```python
from build123d import *

# Parameters (mm, degrees)
EXTRUDE_1_DEPTH     = 100
CUT_EXTRUDE_1_DEPTH = 100


with BuildPart() as part:
    # Model → Бобышка-Вытянуть1 (new body)
    with BuildSketch(Plane.XY):
        with BuildLine():
            Line((-12.5, 11.1), (-12, 11.1))
            Line((-12, 11.1), (-12, 10.6))
            Line((-12, 10.6), (-11.1, 10.6))
            Line((-11.1, 10.6), (-11.1, 13.5))
            Line((-11.1, 13.5), (-9.3, 13.5))
            Line((-9.3, 13.5), (-6.8, 11))
            Line((-6.8, 11), (-6.8, 4))
            Line((-6.8, 4), (-9.3, 1.5))
            Line((-9.3, 1.5), (-11.1, 1.5))
            Line((-11.1, 1.5), (-11.1, 4.4))
            Line((-11.1, 4.4), (-12, 4.4))
            Line((-12, 4.4), (-12, 3.9))
            Line((-12, 3.9), (-12.5, 3.9))
            Line((-12.5, 3.9), (-12.5, 1.5))
            ThreePointArc((-12.5, 1.5), (-12.060660172, 0.439339828), (-11, 0))
            Line((-11, 0), (26.7, 0))
            Line((26.7, 0), (26.7, 1.3))
            Line((26.7, 1.3), (27.5, 1.3))
            Line((27.5, 1.3), (27.5, 6))
            Line((27.5, 6), (22.5, 6))
            Line((22.5, 6), (22.5, 9.9))
            Line((22.5, 9.9), (25.6, 13))
            Line((25.6, 13), (39.4, 13))
            Line((39.4, 13), (42.5, 9.9))
            Line((42.5, 9.9), (42.5, 6))
            Line((42.5, 6), (37.5, 6))
            Line((37.5, 6), (37.5, 1.3))
            Line((37.5, 1.3), (38.3, 1.3))
            Line((38.3, 1.3), (38.3, 0))
            Line((38.3, 0), (71.7, 0))
            Line((71.7, 0), (71.7, 1.3))
            Line((71.7, 1.3), (72.5, 1.3))
            Line((72.5, 1.3), (72.5, 6))
            Line((72.5, 6), (67.5, 6))
            Line((67.5, 6), (67.5, 9.9))
            Line((67.5, 9.9), (70.6, 13))
            Line((70.6, 13), (84.4, 13))
            Line((84.4, 13), (87.5, 9.9))
            Line((87.5, 9.9), (87.5, 6))
            Line((87.5, 6), (82.5, 6))
            Line((82.5, 6), (82.5, 1.3))
            Line((82.5, 1.3), (83.3, 1.3))
            Line((83.3, 1.3), (83.3, 0))
            Line((83.3, 0), (116.7, 0))
            Line((116.7, 0), (116.7, 1.3))
            Line((116.7, 1.3), (117.5, 1.3))
            Line((117.5, 1.3), (117.5, 6))
            Line((117.5, 6), (112.5, 6))
            Line((112.5, 6), (112.5, 9.9))
            Line((112.5, 9.9), (115.6, 13))
            Line((115.6, 13), (129.4, 13))
            Line((129.4, 13), (132.5, 9.9))
            Line((132.5, 9.9), (132.5, 6))
            Line((132.5, 6), (127.5, 6))
            Line((127.5, 6), (127.5, 1.3))
            Line((127.5, 1.3), (128.3, 1.3))
            Line((128.3, 1.3), (128.3, 0))
            Line((128.3, 0), (166, 0))
            ThreePointArc((166, 0), (167.060660172, 0.439339828), (167.5, 1.5))
            Line((167.5, 1.5), (167.5, 3.9))
            Line((167.5, 3.9), (167, 3.9))
            Line((167, 3.9), (167, 4.4))
            Line((167, 4.4), (166.1, 4.4))
            Line((166.1, 4.4), (166.1, 1.5))
            Line((166.1, 1.5), (164.3, 1.5))
            Line((164.3, 1.5), (161.8, 4))
            Line((161.8, 4), (161.8, 11))
            Line((161.8, 11), (164.3, 13.5))
            Line((164.3, 13.5), (166.1, 13.5))
            Line((166.1, 13.5), (166.1, 10.6))
            Line((166.1, 10.6), (167, 10.6))
            Line((167, 10.6), (167, 11.1))
            Line((167, 11.1), (167.5, 11.1))
            Line((167.5, 11.1), (167.5, 13.5))
            ThreePointArc((167.5, 13.5), (167.060660172, 14.560660172), (166, 15))
            Line((166, 15), (150.8, 15))
            Line((150.8, 15), (150.8, 13.7))
            Line((150.8, 13.7), (150, 13.7))
            Line((150, 13.7), (150, 9))
            Line((150, 9), (155, 9))
            Line((155, 9), (155, 5.1))
            Line((155, 5.1), (151.9, 2))
            Line((151.9, 2), (138.1, 2))
            Line((138.1, 2), (135, 5.1))
            Line((135, 5.1), (135, 9))
            Line((135, 9), (140, 9))
            Line((140, 9), (140, 13.7))
            Line((140, 13.7), (139.2, 13.7))
            Line((139.2, 13.7), (139.2, 15))
            Line((139.2, 15), (105.8, 15))
            Line((105.8, 15), (105.8, 13.7))
            Line((105.8, 13.7), (105, 13.7))
            Line((105, 13.7), (105, 9))
            Line((105, 9), (110, 9))
            Line((110, 9), (110, 5.1))
            Line((110, 5.1), (106.9, 2))
            Line((106.9, 2), (93.1, 2))
            Line((93.1, 2), (90, 5.1))
            Line((90, 5.1), (90, 9))
            Line((90, 9), (95, 9))
            Line((95, 9), (95, 13.7))
            Line((95, 13.7), (94.2, 13.7))
            Line((94.2, 13.7), (94.2, 15))
            Line((94.2, 15), (60.8, 15))
            Line((60.8, 15), (60.8, 13.7))
            Line((60.8, 13.7), (60, 13.7))
            Line((60, 13.7), (60, 9))
            Line((60, 9), (65, 9))
            Line((65, 9), (65, 5.1))
            Line((65, 5.1), (61.9, 2))
            Line((61.9, 2), (48.1, 2))
            Line((48.1, 2), (45, 5.1))
            Line((45, 5.1), (45, 9))
            Line((45, 9), (50, 9))
            Line((50, 9), (50, 13.7))
            Line((50, 13.7), (49.2, 13.7))
            Line((49.2, 13.7), (49.2, 15))
            Line((49.2, 15), (15.8, 15))
            Line((15.8, 15), (15.8, 13.7))
            Line((15.8, 13.7), (15, 13.7))
            Line((15, 13.7), (15, 9))
            Line((15, 9), (20, 9))
            Line((20, 9), (20, 5.1))
            Line((20, 5.1), (16.9, 2))
            Line((16.9, 2), (3.1, 2))
            Line((3.1, 2), (0, 5.1))
            Line((0, 5.1), (0, 9))
            Line((0, 9), (5, 9))
            Line((5, 9), (5, 13.7))
            Line((5, 13.7), (4.2, 13.7))
            Line((4.2, 13.7), (4.2, 15))
            Line((4.2, 15), (-11, 15))
            ThreePointArc((-11, 15), (-12.060660172, 14.560660172), (-12.5, 13.5))
            Line((-12.5, 13.5), (-12.5, 11.1))
        make_face()
    extrude(amount=EXTRUDE_1_DEPTH)

    # Эскиз1 → Вырез-Вытянуть1 (cut)
    with BuildSketch(Plane.XY.offset(100)):
        Polygon((-6.8, 7.853553391), (-6.446446609, 7.5), (-6.8, 7.146446609), align=None)
        Polygon((9.646446609, 2), (10, 1.646446609), (10.353553391, 2), align=None)
        Polygon((32.146446609, 13), (32.5, 13.353553391), (32.853553391, 13), align=None)
        Polygon((54.646446609, 2), (55, 1.646446609), (55.353553391, 2), align=None)
        Polygon((77.146446609, 13), (77.5, 13.353553391), (77.853553391, 13), align=None)
        Polygon((99.646446609, 2), (100, 1.646446609), (100.353553391, 2), align=None)
        Polygon((122.146446609, 13), (122.5, 13.353553391), (122.853553391, 13), align=None)
        Polygon((144.646446609, 2), (145, 1.646446609), (145.353553391, 2), align=None)
        Polygon((161.8, 7.853553391), (161.446446609, 7.5), (161.8, 7.146446609), align=None)
    extrude(amount=-CUT_EXTRUDE_1_DEPTH, mode=Mode.SUBTRACT)


solid = part.part
```
Can you work these out from the model? Positions are in its coordinate system, mm. A direction names the side the tool comes from. Coordinates: 2 decimals unless noted, no trailing zeros. Loops run counter-clockwise (first coordinate to the right, second up) from the corner with the lowest first, then second, coordinate; pieces in that order, holes last.
1) For pin 1 (1 mm diameter, centred on y = 14.5, z = 44.5, fed in from -X); pin 2 (1 mm diameter, centred on y = 4.5, z = 84, fed in from -X); pin 3 (0.7 mm diameter, centred on y = 14.5, z = 26, fed in from +X), each with a flat end and sliding along its axis, tell me the tip position at first contact or that it passes through.
2) Imagine slicing it at A-A on x = 102.5. List the corners of the cut face in (y, z) for me, plus the area to 3 significant figures.
3) Which directions (+Z, -Z, +X, -X, +Y, -Y) give clear straight access to the entire face, cutting with the end or side of a thin tool? Please do faces 5 (the flat face through (105, 11, 49)), 6 (the flat face through (40.9, 11.5, 49.3)), 7 (the flat face through (127.5, 4, 49)).
4) Thinking about a two-plate mould opening in Y: for faces 1 (the flat face through (33, 15, 49)), 2 (the flat face through (45, 7, 49)), 3 (the flat face through (42.5, 8, 49)), 4 (the flat face through (5, 11, 49)), which applies, pulls with the +Y half, pulls with the -Y half, needs draft (parallel to the pull), parting line crosses it, or undercut?
5) I need wall thicknesses on probe 1 along X at (y, z) = (14.5, 79); probe 2 along Y at (x, z) = (117, 30.5); probe 3 along Y at (x, z) = (115, 81.5). Which ranges of each line are inside material? Lowest first, please.
Completed:
1. pin 1: stops at x = -12.41
1. pin 2: stops at x = -12
1. pin 3: stops at x = 167.35
2. outline: (0, 0) - (2, 0) - (2, 100) - (0, 100) - close
2. area: 200 mm2
3. face 5: +Z, -Z, +Y
3. face 6: +Z, -Z
3. face 7: +Z, -Z, -Y
4. face 1: pulls with the +Y half
4. face 2: undercut
4. face 3: undercut
4. face 4: needs draft
5. probe 1: x = -12.12 to 4.2, 15.8 to 49.2, 60.8 to 94.2, 105.8 to 139.2, 150.8 to 167.12
5. probe 2: y = 1.3 to 6, 13 to 15
5. probe 3: y = 0 to 6, 12.4 to 15
